Build history of the part. All positions in model axes, mm. A direction names the side the tool comes from. Round coordinates to 2 decimals unless told otherwise and drop trailing zeros. Write each loop counter-clockwise with the first axis right and the second up, starting at its lowest first coordinate (ties: lowest second). Pieces come first, ordered by that corner, then holes. Notation, with made-up numbers: M 28,-20.75 L 36,-20.75 A15 ccw 36,4.25 Z; hole C 29,38 d11. An arc over 180 degrees is marked long. Write item = value, one per line. Start each with the question number.
Q1. Pull direction Z, two halves, no side cores. Call faces 1 (the flat face through (222, -39, 0)), 2 (the flat face through (44.7, -39.3, 18.8)), 3 (the flat face through (254, -39, 31)): released by +Z, released by -Z, zero draft, split by the parting line, or undercut.
Q2. Band-saw the part on D-D on y = -80. Write the cut outline in (x, z).
Q3. Band-saw the part on C-C on x = 83. Write the cut outline in (y, z), plus the area to 3 significant figures.
Q4. Probe L1, parallel to Z at x = 238.5, y = -48; L2, parallel to Z at x = 113.5, y = -43.5; L3, parallel to X at y = 4, z = 154. List the from-to ranges inside material, lowest first.
Q5. Band-saw the part on B-B on z = 124. Write the cut outline in (x, y), plus the area to 3 significant figures.
Q6. Band-saw the part on A-A on y = -11. Write the cut outline in (x, z).
Q7. Tool access for faces 4 (the flat face through (145, 0, 66)), 5 (the flat face through (126, -39, 38.1)), 6 (the flat face through (166, -25.4, 117)), 7 (the flat face through (129, -63, 63.5)), 8 (the cylindrical face through (215.61, -12.52, 169.59)): list every direction of +Z, -Z, +X, -X, +Y, -Y with a clear straight run to the whole face (end or side of a thin tool).
Q8. Drop flat-ended pins along their axis: P1, Ø2, axis at x = 116.5, y = -53, coming from the -Z side; P2, Ø5, axis at x = 123, y = -105, coming from the +Z side; P3, Ø1.5, axis at y = 6.5, z = 166.5, coming from the +X side; P4, Ø1, axis at y = -26, z = 212.5, coming from the +X side. Give the stop position or say it passes through.
```python
from build123d import *

# Parameters (mm, degrees)
F1_DEPTH = 127
F0_R     = 50.8
F2_DEPTH = 50.8
F3_DEPTH = 25.4


with BuildPart() as f1:
    # F0 (on Front) → F1 (new body)
    with BuildSketch(Plane.XZ):
        Polygon((0, 63.5), (0, 0), (63.5, 0), (25.4, 38.1), (63.5, 38.1), (190.5, 38.1), (228.6, 38.1), (190.5, 0), (254, 0), (254, 63.5), align=None)
    extrude(amount=F1_DEPTH)

    # F0 (on Front) → F2 (join)
    with BuildSketch(Plane.XZ):
        with BuildLine():
            Line((44.395084, 185.368859), (0, 63.5))
            Line((0, 63.5), (254, 63.5))
            Line((254, 63.5), (211.859648, 184.235612))
            ThreePointArc((211.859648, 184.235612), (215.575085, 169.796736), (216.825286, 154.94))
            ThreePointArc((216.825286, 154.94), (112.47577, 67.392742), (44.395084, 185.368859))
        make_face()
        with BuildLine():
            ThreePointArc((211.859648, 184.235612), (128.526866, 243.837965), (44.395084, 185.368859))
            ThreePointArc((44.395084, 185.368859), (112.47577, 67.392742), (216.825286, 154.94))
            ThreePointArc((216.825286, 154.94), (215.575085, 169.796736), (211.859648, 184.235612))
        make_face()
        with Locations((127.925286, 154.94)):
            Circle(F0_R, mode=Mode.SUBTRACT)
        Polygon((0, 63.5), (0, 0), (63.5, 0), (25.4, 38.1), (63.5, 38.1), (190.5, 38.1), (228.6, 38.1), (190.5, 0), (254, 0), (254, 63.5), align=None)
    extrude(amount=-F2_DEPTH)

    # F0 (on Front) → F3 (join)
    with BuildSketch(Plane.XZ):
        with BuildLine():
            ThreePointArc((211.859648, 184.235612), (128.526866, 243.837965), (44.395084, 185.368859))
            ThreePointArc((44.395084, 185.368859), (112.47577, 67.392742), (216.825286, 154.94))
            ThreePointArc((216.825286, 154.94), (215.575085, 169.796736), (211.859648, 184.235612))
        make_face()
        with Locations((127.925286, 154.94)):
            Circle(F0_R, mode=Mode.SUBTRACT)
    extrude(amount=F3_DEPTH)


solid = f1.part
```
Conclusion:
q1.face_1 = released by -Z
q1.face_2 = undercut
q1.face_3 = zero draft
q2.outline = M 0,0 L 63.5,0 L 25.4,38.1 L 228.6,38.1 L 190.5,0 L 254,0 L 254,63.5 L 0,63.5 Z
q3.outline = M -127,38.1 L 50.8,38.1 L 50.8,131.23 L -25.4,131.23 L -25.4,78.23 L 0,78.23 L 0,63.5 L -127,63.5 Z; M -25.4,178.65 L 50.8,178.65 L 50.8,231.65 L -25.4,231.65 Z
q3.area = 13,300 mm^2
q4.L1 = 0 to 63.5
q4.L2 = 38.1 to 63.5
q4.L3 = 32.97 to 77.13, 178.72 to 222.41
q5.outline = M 22.04,0 L 44.58,0 L 44.58,-25.4 L 87.63,-25.4 L 87.63,50.8 L 22.04,50.8 Z; M 168.22,-25.4 L 211.27,-25.4 L 211.27,0 L 232.88,0 L 232.88,50.8 L 168.22,50.8 Z
q5.area = 8,800 mm^2
q6.outline = M 0,0 L 63.5,0 L 25.4,38.1 L 228.6,38.1 L 190.5,0 L 254,0 L 254,63.5 L 0,63.5 Z; M 211.86,184.24 A88.9 ccw long 216.83,154.94 A88.9 ccw Z; hole C 127.93,154.94 d101.6
q7.face_4 = -Y
q7.face_5 = +Y, -Y
q7.face_6 = +Z, +X, -X, -Y
q7.face_7 = +X, -X, -Y
q7.face_8 = +Z, +X, -Y
q8.P1 = 38.1
q8.P2 = 63.5
q8.P3 = 218.31
q8.P4 = through
